The listing builds one solid part. Answer for the finished solid, in the listing's coordinates (mm). A direction names the side the tool comes from. Give positions to 0.01 mm unless a question says otherwise; leave off trailing zeros. Order: outer loops, then holes, each group sorted by start corner. A loop starts at its lowest first (then second) coordinate and runs counter-clockwise, first axis right, second up. Notation, with made-up numbers: M 5.5,12 L 43.5,12 A13 ccw 43.5,36 Z; hole C 26,-1.75 d11. An arc over 180 degrees is marked long. Answer as a JSON object with one key per item and string values. Group by question number.
```python
from build123d import *

# Parameters (mm, degrees)
SKETCH1_W           = 21.825
SKETCH1_H           = 3.175
SKETCH1_W_2         = 3.175
SKETCH1_H_2         = 20.5
BOSS_EXTRUDE1_DEPTH = 3.175
SKETCH2_W           = 5
SKETCH2_H           = 26
SKETCH2_W_2         = 10
SKETCH2_H_2         = 3.175
CUT_EXTRUDE1_DEPTH  = 23.175


with BuildPart() as part:
    # Sketch1 → Boss-Extrude1 (new body)
    with BuildSketch(Plane(origin=(0, 0, 0), x_dir=(1, 0, 0), z_dir=(0, 1, 0))):
        Polygon((-20, 31.825), (-41.825, 31.825), (-41.825, -7.25), (-41.825, -27.75), (-41.825, -31.825), (-20, -31.825), (20, -31.825), (41.825, -31.825), (41.825, -27.75), (41.825, -7.25), (41.825, 31.825), (20, 31.825), align=None)
        with Locations((30.9125, 33.4125)):
            Rectangle(SKETCH1_W, SKETCH1_H)
        with Locations((-30.9125, 33.4125)):
            Rectangle(SKETCH1_W, SKETCH1_H)
        with Locations((-43.4125, -17.5)):
            Rectangle(SKETCH1_W_2, SKETCH1_H_2)
        with Locations((43.4125, -17.5)):
            Rectangle(SKETCH1_W_2, SKETCH1_H_2)
    extrude(amount=BOSS_EXTRUDE1_DEPTH)

    # Sketch2 → Cut-Extrude1 (cut)
    with BuildSketch(Plane(origin=(0, 3.175, 0), x_dir=(1, 0, 0), z_dir=(0, 1, 0))):
        with Locations((-35.325, -15.5)):
            Rectangle(SKETCH2_W, SKETCH2_H)
        with Locations((35.325, -15.5)):
            Rectangle(SKETCH2_W, SKETCH2_H)
        with Locations((-18.075, -3.9125)):
            Rectangle(SKETCH2_W_2, SKETCH2_H_2)
        with Locations((18.075, -3.9125)):
            Rectangle(SKETCH2_W_2, SKETCH2_H_2)
        with Locations((18.075, -27.0875)):
            Rectangle(SKETCH2_W_2, SKETCH2_H_2)
        with Locations((-18.075, -27.0875)):
            Rectangle(SKETCH2_W_2, SKETCH2_H_2)
    extrude(amount=-CUT_EXTRUDE1_DEPTH, mode=Mode.SUBTRACT)


solid = part.part
```
Item 1: Flat-ended cylindrical pins translate along their axes: P1, Ø1, axis at x = 43, y = 1, coming from the -Z side; P2, Ø1.6, axis at y = 2, z = -34, coming from the -X side (3 decimals); P3, Ø1, axis at y = 1.5, z = -34, coming from the +X side (3 decimals); P4, Ø4, axis at x = -1, z = 6.5, coming from the -Y side. Find the tip coordinate at first contact, or state that the pin passes through.
Item 2: A tool of negligible diameter and unlimited length cuts with its end or side. For faces 5 (the flat face through (45, 2, 18)), 6 (the flat face through (23.075, 2, 4)), 7 (the flat face through (-43, 2, 7.25)), 8 (the flat face through (-20, 2, -33)), 9 (the flat face through (41.825, 2, 30)), from which of +Z, -Z, +X, -X, +Y, -Y can it reach the whole face along a straight path? Write none if from no direction.
Item 3: Section D-D (z = -30) is taken. Determine the outline of the cut face in (x, y) (3 decimals), and give its area (3 significant figures).
Item 4: Consider probe 1 along X at (y, z) = (1.3, 7.5) (3 decimals); probe 2 along Z at (x, y) = (-15, 2.3) (3 decimals); probe 3 along Z at (x, y) = (22, 2.65) (3 decimals). Determine where each line is inside the solid, lowest interval first. Write a range as from..to.
Item 5: Section A-A (z = 9) is taken. Determine the outline of the cut face in (x, y) (3 decimals).
Item 6: Determine the mould class of faces 1 (the flat face through (-1, 3.175, -2)), 2 (the flat face through (32.825, 2, 16)), 3 (the flat face through (43, 2, 27.75)), 4 (the flat face through (-18, 2, 28.675)) for opening direction Z: released by +Z, released by -Z, zero draft, split by the parting line, or undercut.
Item 7: Section C-C (x = -9.5) is taken. Determine the outline of the cut face in (y, z) (3 decimals).
Item 8: Section B-B (y = 1) is taken. Count the separate pieces of the cut face and the enclosed holes in it, and give its area (3 significant figures).
Values found:
{
 "1": {"P1": "stops at z = 7.25", "P2": "stops at x = -41.825", "P3": "stops at x = 41.825", "P4": "stops at y = 0"},
 "2": {"face 5": "+Z, -Z, +X, +Y, -Y", "face 6": "+Y, -Y", "face 7": "-Z, -X, +Y, -Y", "face 8": "-Z, +Y, -Y", "face 9": "+Z, +X, +Y, -Y"},
 "3": {"outline": "M -41.825,0 L 41.825,0 L 41.825,3.175 L -41.825,3.175 Z", "area": "266 mm^2"},
 "4": {"probe 1": "x = -45..-37.825, -32.825..32.825, 37.825..45", "probe 2": "z = -31.825..2.325, 5.5..25.5, 28.675..31.825", "probe 3": "z = -35..2.325, 5.5..25.5, 28.675..31.825"},
 "5": {"outline": "M -45,0 L -37.825,0 L -37.825,3.175 L -45,3.175 Z; M -32.825,0 L 32.825,0 L 32.825,3.175 L -32.825,3.175 Z; M 37.825,0 L 45,0 L 45,3.175 L 37.825,3.175 Z"},
 "6": {"face 1": "zero draft", "face 2": "undercut", "face 3": "released by +Z", "face 4": "undercut"},
 "7": {"outline": "M 0,-31.825 L 3.175,-31.825 L 3.175,31.825 L 0,31.825 Z"},
 "8": {"separate pieces": "1", "enclosed holes": "6", "area": "5,210 mm^2"}
}
